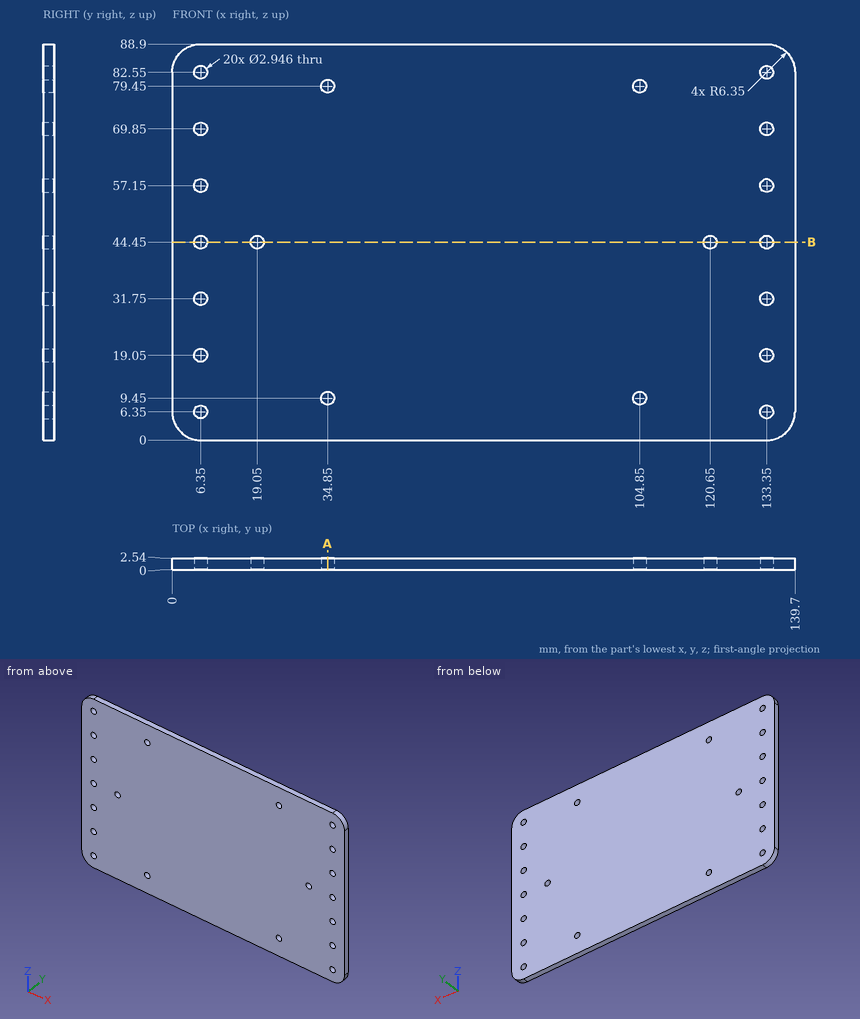
Check sheet for the drawn part. Datum: minimum x, y, z corner. Units: mm. Round coordinates to 2 decimals unless told otherwise and drop trailing zeros. Loops run counter-clockwise (first coordinate to the right, second up) from the corner with the lowest first, then second, coordinate; pieces in that order, holes last.
Item 1: Gauge pin test, flat end, axial feed: pin 1 (2.5 mm diameter, centred on x = 133.35, z = 6.35, fed in from +Y). Record the tip position at first contact, or that the pin passes through.
Item 2: Cross-section at B-B on z = 44.45. Record the boundary of the cut face in (x, y), then the cut area to 3 significant figures.
Item 3: Cross-section at A-A on x = 34.85. Record the boundary of the cut face in (y, z), then the cut area to 3 significant figures.
Item 4: Thickness scan on line 1 (X direction, y = 0.7, z = 44.45); line 2 (X direction, y = 0.75, z = 69.85); line 3 (X direction, y = 1.95, z = 56.5). Record the ranges inside material, lowest first.
Answer sheet:
1. pin 1: passes through
2. outline: (0, 0) - (4.88, 0) - (4.88, 2.54) - (0, 2.54) - close; (7.82, 0) - (17.58, 0) - (17.58, 2.54) - (7.82, 2.54) - close; (20.52, 0) - (119.18, 0) - (119.18, 2.54) - (20.52, 2.54) - close; (122.12, 0) - (131.88, 0) - (131.88, 2.54) - (122.12, 2.54) - close; (134.82, 0) - (139.7, 0) - (139.7, 2.54) - (134.82, 2.54) - close
2. area: 325 mm2
3. outline: (0, 0) - (2.54, 0) - (2.54, 7.98) - (0, 7.98) - close; (0, 10.92) - (2.54, 10.92) - (2.54, 77.98) - (0, 77.98) - close; (0, 80.92) - (2.54, 80.92) - (2.54, 88.9) - (0, 88.9) - close
3. area: 211 mm2
4. line 1: x = 0 to 4.88, 7.82 to 17.58, 20.52 to 119.18, 122.12 to 131.88, 134.82 to 139.7
4. line 2: x = 0 to 4.88, 7.82 to 131.88, 134.82 to 139.7
4. line 3: x = 0 to 5.03, 7.67 to 132.03, 134.67 to 139.7
